Autodesk Inventor part; units mm, degrees
ref_plane "YZ Plane" through (0, 0, 0) normal (1, 0, 0) x (0, 1, 0)
ref_plane "XZ Plane" through (0, 0, 0) normal (0, 1, 0) x (-1, 0, 0)
ref_plane "XY Plane" through (0, 0, 0) normal (0, 0, 1) x (1, 0, 0)
sketch "Sketch1" plane through (0, 0, 0) normal (0, 1, 0) x (-1, 0, 0)
  circle A0 centre (0, 0) radius 32.5
  circle A1 centre (0, 0) radius 35.5
  dimension "d0" = 65
  dimension "d1" = 71
extrude "Extrusion1" add sketch "Sketch1" along normal blind 10
extrude "Extrusion2" add sketch "Sketch1" along normal blind 3 contours A0
sketch "Sketch2" plane through (0, 3, 0) normal (0, 1, 0) x (1, 0, 0)
  circle A0 centre (0, 0) radius 32.5
  line L0 (0, 32.5) -> (0, 29.5)
  line L1 (-1.5, 29.5) -> (-1.5, 32.5)
  line L2 (-1.5, 32.5) -> (1.5, 32.5)
  line L3 (1.5, 32.5) -> (1.5, 29.5)
  line L4 (1.5, 29.5) -> (-1.5, 29.5)
  line L5 (-1.5, 29.5) -> (1.5, 32.5) construction
  line L6 (-1.5, 32.5) -> (1.5, 29.5) construction
  point P0 (0, 31)
  point P1 (1.5, 32.4654)
  point P2 (-1.5, 32.4654)
  dimension "d7" = 3
  dimension "d8" = 3
extrude "Extrusion3" add sketch "Sketch2" along normal blind 2.5 contours L3 L4 L0 A0 | A0 L0 L4 L1
pattern_circular "Circular Pattern1" count 3 over 360 about axis through (0, -10, 0) along (0, 1, 0) of "Extrusion3"
properties part number "Orchid Coaster V1"
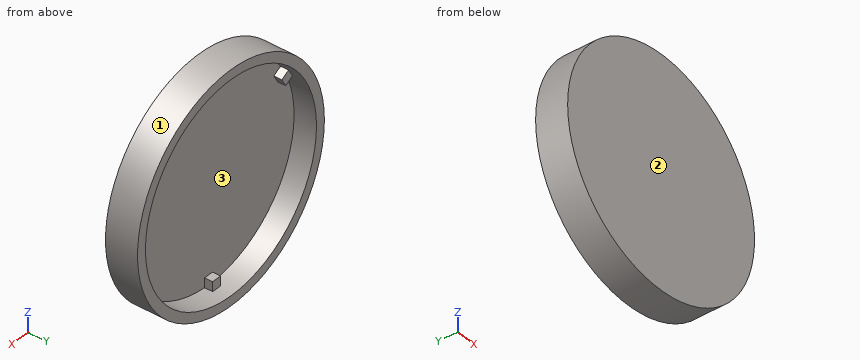
Work out the finished part from the listing and answer in its coordinate system (mm). Face numbers are marked on the shaded views. Round coordinates to 2 decimals unless told otherwise and drop trailing zeros. Order: outer loops, then holes, each group sorted by start corner. A loop starts at its lowest first (then second) coordinate and runs counter-clockwise, first axis right, second up. Notation, with made-up numbers: M 80,26 L 84,26 A6 ccw 84,37 Z; hole C 65.5,-15 d4. An arc over 180 degrees is marked long. One line per item, written item: value.
Q1. Find section A-A on x = 0. Write down the section's boundary in (y, z).
Derived:
outline: M 0,-35.5 L 10,-35.5 L 10,-32.5 L 5.5,-32.5 L 5.5,-29.5 L 3,-29.5 L 3,32.5 L 10,32.5 L 10,35.5 L 0,35.5 Z
Q2. Determine the mould class of the marked faces 1, 2 and 3 for opening direction Z: released by +Z, released by -Z, zero draft, split by the parting line, or undercut.
Derived:
face 1: split by the parting line
face 2: zero draft
face 3: undercut
Q3. Find section B-B on z = -21.5. Write down the section's boundary in (x, y), then the cut area to 3 significant figures.
Derived:
outline: M -28.25,0 L 28.25,0 L 28.25,10 L 24.37,10 L 24.37,3 L -24.37,3 L -24.37,10 L -28.25,10 Z
area: 224 mm²
Q4. Straight lines are drawn through the part: line 1 (Z direction, x = 0, y = 4.75); line 2 (X direction, y = 7.5, z = 0.5); line 3 (Y direction, x = -16, z = 27). For each, find the intervals that lie inside material, in ascending order.
Derived:
line 1: -35.5 to -29.5, 32.5 to 35.5
line 2: -35.5 to -32.5, 32.5 to 35.5
line 3: 0 to 3
Q5. Flat-ended cylindrical pins translate along their axes: pin 1 (3 mm diameter, centred on x = 0.5, y = 4.5, fed in from +Z); pin 2 (10 mm diameter, centred on x = 7.5, z = 7.5, fed in from -Y); pin 3 (1.5 mm diameter, centred on x = -4.5, y = 4.5, fed in from -Z); pin 4 (19.5 mm diameter, centred on x = -5.5, z = 8, fed in from +Y). Find the tip coordinate at first contact, or state that the pin passes through.
Derived:
pin 1: z = 35.5
pin 2: y = 0
pin 3: z = -35.3
pin 4: y = 3
Q6. Find section D-D on x = 19. Write down the section's boundary in (y, z), then the cut area to 3 significant figures.
Derived:
outline: M 0,-29.99 L 10,-29.99 L 10,-26.37 L 3,-26.37 L 3,26.37 L 10,26.37 L 10,29.99 L 0,29.99 Z
area: 231 mm²
Q7. Find section C-C on y = 6.5. Write down the section's boundary in (x, z), then the cut area to 3 significant figures.
Derived:
outline: C 0,0 d71; hole C 0,0 d65
area: 641 mm²
